```python
from build123d import *

# Parameters (mm, degrees)
F0_W      = 101.3216488063
F0_H      = 117.805339396
F1_DEPTH  = 145.796
F2_W      = 145.796
F2_H      = 117.805339396
F3_DEPTH  = 89.916
F4_W      = 168.2205758989
F4_H      = 121.5348821133
F5_DEPTH  = 153.924
F6_SIZE   = 5.08
F7_W      = 145.796
F7_H      = 117.805339396
F8_DEPTH  = 254.508
F9_W      = 145.796
F9_H      = 117.805339396
F10_DEPTH = 254.508
F11_W     = 143.2336866856
F11_H     = 104.3559815735
F11_W_2   = 141.1875188351
F11_H_2   = 107.7663134784
F12_DEPTH = 95.758
F13_SIZE  = 5.08
F14_R     = 52.2748523049
F15_DEPTH = 281.686


with BuildPart() as f1:
    # F0 (on Front) → F1 (new body)
    with BuildSketch(Plane.XZ):
        with Locations((-1.7741117626, -7.8057236969)):
            Rectangle(F0_W, F0_H)
    extrude(amount=F1_DEPTH)

    # F2 (on face) → F3 (join)
    with BuildSketch(Plane.YZ.offset(48.8867126405)):
        with Locations((-72.898, -7.8057236969)):
            Rectangle(F2_W, F2_H)
    extrude(amount=F3_DEPTH)

    # F4 (on face) → F5 (join)
    with BuildSketch(Plane.XY.offset(51.0969460011)):
        with Locations((40.545957163, -71.0269669071)):
            Rectangle(F4_W, F4_H)
    extrude(amount=F5_DEPTH)

    # F6
    f6_edges = [f1.edges().sort_by_distance(p)[0] for p in [
        (40.545957, -131.794408, 205.020946),
        (124.656245, -71.026967, 205.020946),
        (40.545957, -10.259526, 205.020946),
        (-43.564331, -71.026967, 205.020946),
    ]]
    chamfer(f6_edges, length=F6_SIZE)

    # F7 (on face) → F8 (join)
    with BuildSketch(Plane.YZ.offset(138.8027126405)):
        with Locations((-72.898, -7.8057236969)):
            Rectangle(F7_W, F7_H)
    extrude(amount=F8_DEPTH)

    # F9 (on face) → F10 (join)
    with BuildSketch(Plane(origin=(-52.4349361658, 0, 0), x_dir=(0, -1, 0), z_dir=(-1, 0, 0))):
        with Locations((72.898, -7.8057236969)):
            Rectangle(F9_W, F9_H)
    extrude(amount=F10_DEPTH)

    # F11 (on face) → F12 (join)
    with BuildSketch(Plane.XY.offset(51.0969460011)):
        with Locations((-185.3079646826, -68.4645744041)):
            Rectangle(F11_W, F11_H)
        with Locations((271.3347226381, -70.1697403565)):
            Rectangle(F11_W_2, F11_H_2)
    extrude(amount=F12_DEPTH)

    # F13
    f13_edges = [f1.edges().sort_by_distance(p)[0] for p in [
        (-185.307965, -16.286584, 146.854946),
        (-113.691121, -68.464574, 146.854946),
        (-185.307965, -120.642565, 146.854946),
        (-256.924808, -68.464574, 146.854946),
        (271.334723, -16.286584, 146.854946),
        (200.740963, -70.16974, 146.854946),
        (341.928482, -70.16974, 146.854946),
        (271.334723, -124.052897, 146.854946),
    ]]
    chamfer(f13_edges, length=F13_SIZE)

    # F14 (on face) → F15 (join)
    with BuildSketch(Plane.XY.offset(205.0209460011)):
        with Locations((44.2011877894, -70.0180381536)):
            Circle(F14_R)
    extrude(amount=F15_DEPTH)


solid = f1.part
```
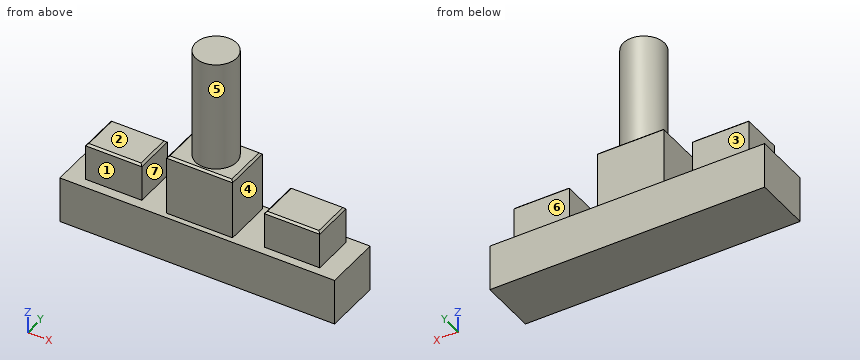
Work out the finished part from the listing and answer in its coordinate system (mm). Face numbers are marked on the shaded views. A direction names the side the tool comes from. Round coordinates to 2 decimals unless told otherwise and drop trailing zeros. Write each loop counter-clockwise with the first axis right and the second up, starting at its lowest first coordinate (ties: lowest second). Pieces come first, ordered by that corner, then holes. Notation, with made-up numbers: (60.25, 81.5) -> (100.25, 81.5) arc R17 cw to (100.25, 107.5) -> close; hole circle Ø4 at (35.25, -28.5). An arc over 180 degrees is marked (long way). Write each question's results on one line, items separated by ' | '.
Q1. Section C-C, the plane y = -100 is taken. Write down the section's boundary in (x, z), then the cut area to 3 significant figures.
Data:
outline: (-306.94, -66.71) -> (393.31, -66.71) -> (393.31, 51.1) -> (341.93, 51.1) -> (341.93, 141.77) -> (336.85, 146.85) -> (205.82, 146.85) -> (200.74, 141.77) -> (200.74, 51.1) -> (124.66, 51.1) -> (124.66, 199.94) -> (119.58, 205.02) -> (87.02, 205.02) -> (87.02, 486.71) -> (1.38, 486.71) -> (1.38, 205.02) -> (-38.48, 205.02) -> (-43.56, 199.94) -> (-43.56, 51.1) -> (-113.69, 51.1) -> (-113.69, 141.77) -> (-118.77, 146.85) -> (-251.84, 146.85) -> (-256.92, 141.77) -> (-256.92, 51.1) -> (-306.94, 51.1) -> close | area: 160,000 mm^2
Q2. Section D-D, the plane z = 181 is taken. Write down the section's boundary in (x, y).
Data:
outline: (-43.56, -131.79) -> (124.66, -131.79) -> (124.66, -10.26) -> (-43.56, -10.26) -> close
Q3. Determine the mould class of the marked faces 5, 6 and 7 for opening direction X: released by +X, released by -X, zero draft, split by the parting line, or undercut.
Data:
face 5: split by the parting line | face 6: zero draft | face 7: undercut
Q4. Section A-A, the plane z = 104 is taken. Write down the section's boundary in (x, y), then the cut area to 3 significant figures.
Data:
outline: (-256.92, -120.64) -> (-113.69, -120.64) -> (-113.69, -16.29) -> (-256.92, -16.29) -> close; (-43.56, -131.79) -> (124.66, -131.79) -> (124.66, -10.26) -> (-43.56, -10.26) -> close; (200.74, -124.05) -> (341.93, -124.05) -> (341.93, -16.29) -> (200.74, -16.29) -> close | area: 50,600 mm^2
Q5. Section B-B, the plane x = -148.5 is taken. Write down the section's boundary in (y, z).
Data:
outline: (-145.8, -66.71) -> (0, -66.71) -> (0, 51.1) -> (-16.29, 51.1) -> (-16.29, 141.77) -> (-21.37, 146.85) -> (-115.56, 146.85) -> (-120.64, 141.77) -> (-120.64, 51.1) -> (-145.8, 51.1) -> close
Q6. Which of the six approach directions +Z, -Z, +X, -X, +Y, -Y give full straight-line access (tool end or side, diameter ignored) to the marked faces 1, 2, 3 and 4?
Data:
face 1: +Z, -X, -Y | face 2: +Z, -X, +Y, -Y | face 3: +Z, -X, +Y | face 4: +Z, +Y, -Y
Q7. Straight lines are drawn through the part: line 1 along X through (y, z) = (-54.5, 125); line 2 along Z through (x, y) = (147, -13); line 3 along Y through (x, z) = (-199, 137.5). For each, find the intervals that lie inside material, in ascending order. Write a range as [from, to].
Data:
line 1: [-256.92, -113.69], [-43.56, 124.66], [200.74, 341.93] | line 2: [-66.71, 51.1] | line 3: [-120.64, -16.29]
Q8. Flat-ended cylindrical pins translate along their axes: P1, Ø6, axis at y = -46, z = 75, coming from the +X side; P2, Ø8, axis at x = -1.5, z = 115.5, coming from the +Y side; P3, Ø12, axis at y = -108, z = 333.5, coming from the -X side. Find the tip coordinate at first contact, or state that the pin passes through.
Data:
P1: x = 341.93 | P2: y = -10.26 | P3: x = 2.85
